Verification items for this drawing (mm, ordinates from the low corner). Round coordinates to 2 decimals unless told otherwise and drop trailing zeros. Write each loop counter-clockwise with the first axis right and the second up, starting at its lowest first coordinate (ties: lowest second). Pieces come first, ordered by that corner, then holes.
Item 1: Cross-section at B-B (x = 6.35). Enter the section's corners in (y, z).
Item 2: Cross-section at A-A (z = 6.35). Enter the section's corners in (x, y).
Item 3: Depth check by flat-ended pin: P1, Ø1.5, axis at y = 6, z = 1.5, coming from the +X side; P2, Ø3, axis at y = 4.5, z = 2.5, coming from the -X side; P3, Ø1.5, axis at y = 21, z = 3.5, coming from the -X side; P4, Ø6, axis at x = 6, z = 5.5, coming from the -Y side. Enter the tip coordinate at first touch or a pass-through.
Item 4: Cross-section at C-C (y = 4). Enter the section's corners in (x, z).
Item 5: Cross-section at D-D (x = 9.5). Enter the section's corners in (y, z).
Item 6: Draft check along X on the marked faces 1, 2, 3 and 4. Enter one of: pulls with the +X half, pulls with the -X half, needs draft (parallel to the pull), parting line crosses it, or undercut.
Item 7: Scan lines: probe 1 along X at (y, z) = (15.5, 6.35); probe 2 along X at (y, z) = (6.35, 11.7); probe 3 along Z at (x, y) = (4.5, 4.75) (1 decimal). Record each from-to range of solid material in increasing order.
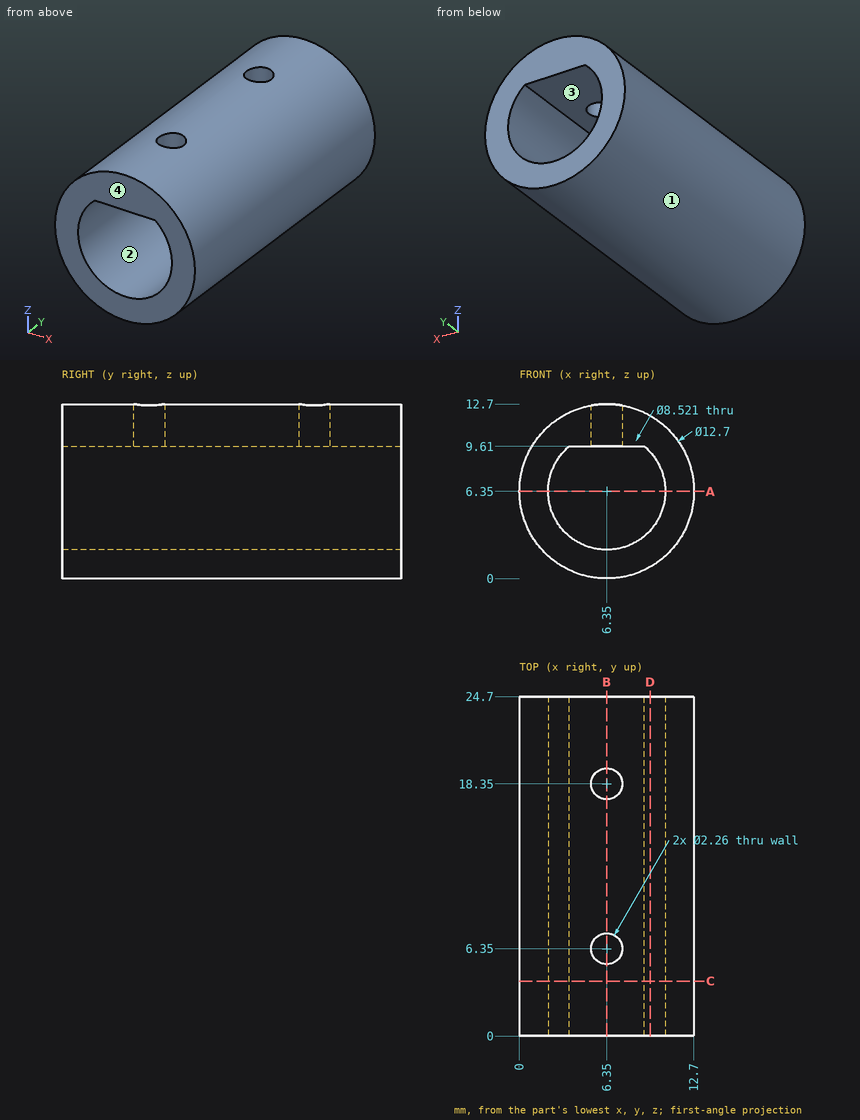
Resolved:
1. outline: (0, 0) - (24.7, 0) - (24.7, 2.09) - (0, 2.09) - close; (0, 9.61) - (5.22, 9.61) - (5.22, 12.7) - (0, 12.7) - close; (7.48, 9.61) - (17.22, 9.61) - (17.22, 12.7) - (7.48, 12.7) - close; (19.48, 9.61) - (24.7, 9.61) - (24.7, 12.7) - (19.48, 12.7) - close
2. outline: (0, 0) - (2.09, 0) - (2.09, 24.7) - (0, 24.7) - close; (10.61, 0) - (12.7, 0) - (12.7, 24.7) - (10.61, 24.7) - close
3. P1: stops at x = 11.2
3. P2: stops at x = 0.45
3. P3: stops at x = 0.36
3. P4: passes through
4. outline: circle Ø12.7 at (6.35, 6.35); hole (3.61, 9.61) arc R4.26 ccw (long way) to (9.09, 9.61) - close
5. outline: (0, 0.84) - (24.7, 0.84) - (24.7, 3.48) - (0, 3.48) - close; (0, 9.22) - (24.7, 9.22) - (24.7, 11.86) - (0, 11.86) - close
6. face 1: parting line crosses it
6. face 2: undercut
6. face 3: undercut
6. face 4: needs draft
7. probe 1: x = 0 to 2.09, 10.61 to 12.7
7. probe 2: x = 2.93 to 5.22, 7.48 to 9.77
7. probe 3: z = 0.3 to 2.5, 9.6 to 12.4
